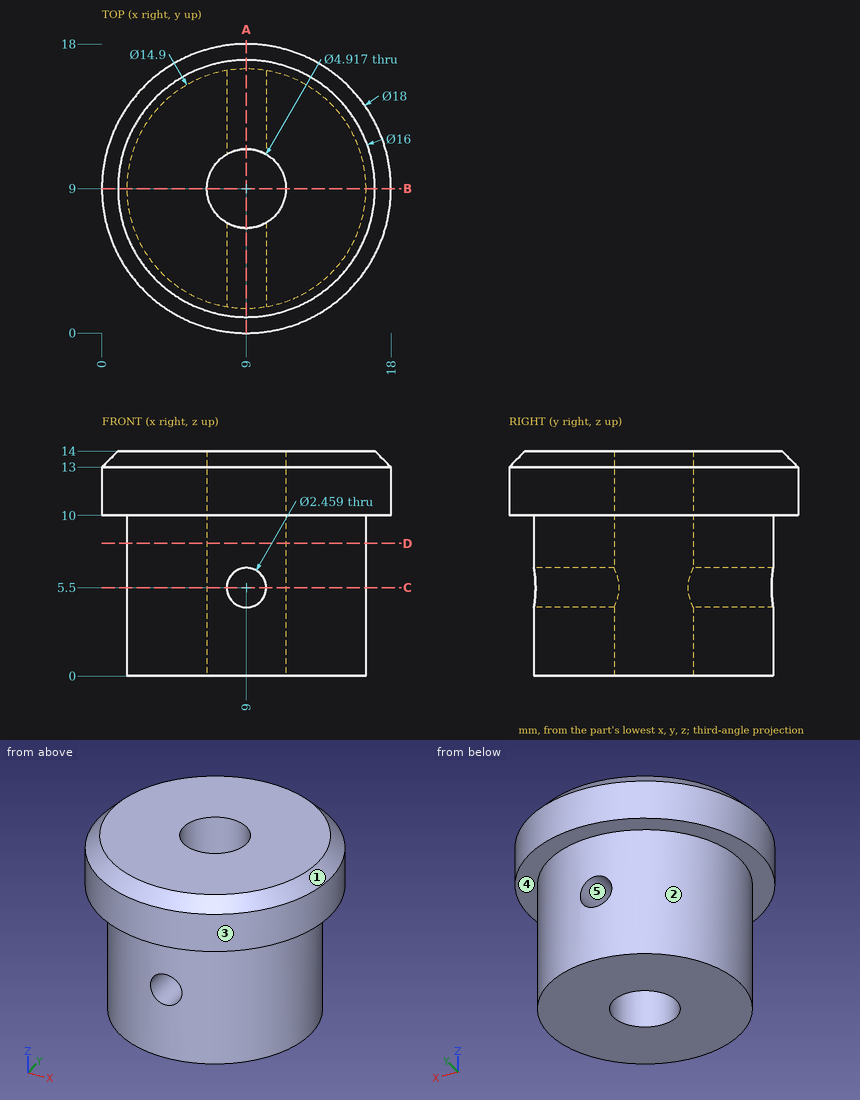
Here's the drawing with two shaded views (mm, measured from the low corner). I have some questions. A direction names the side the tool comes from. Coordinates: 2 decimals unless noted, no trailing zeros. Write each loop counter-clockwise with the first axis right and the second up, starting at its lowest first coordinate (ties: lowest second). Pieces come first, ordered by that corner, then holes. Notation, with made-up numbers: M 10.25,86 L 37.25,86 A26 cw 37.25,110 Z; hole C 21,32 d4. An arc over 180 degrees is marked long. Use one line per item in the form item = value.
Q1. If we section it at C-C (z = 5.5): Write out the boundary of the cut face in (x, y).
Model answer:
outline = M 7.77,1.65 L 7.77,6.87 A2.46 cw 7.77,11.13 L 7.77,16.35 A7.45 ccw Z; M 10.23,1.65 A7.45 ccw 10.23,16.35 L 10.23,11.13 A2.46 cw 10.23,6.87 Z
Q2. I need wall thicknesses on line 1 along Z through (x, y) = (9, 2.6); line 2 along Y through (x, z) = (9, 3); line 3 along Z through (x, y) = (13.25, 15.75). Which ranges of each line are inside material? Lowest first, please. Write a range as from..to.
Model answer:
line_1 = 0..4.27, 6.73..14
line_2 = 1.55..6.54, 11.46..16.45
line_3 = 10..14
Q3. If we section it at B-B (y = 9): Write out the boundary of the cut face in (x, z).
Model answer:
outline = M 0,10 L 1.55,10 L 1.55,0 L 6.54,0 L 6.54,14 L 1,14 L 0,13 Z; M 11.46,0 L 16.45,0 L 16.45,10 L 18,10 L 18,13 L 17,14 L 11.46,14 Z
Q4. For P1, Ø3, axis at x = 9, z = 5.5, coming from the +Y side; P2, Ø3, axis at x = 9, y = 9, coming from the -Z side; P3, Ø8, axis at y = 2.5, z = 4.5, coming from the +X side; P4, Ø1, axis at y = 3.5, z = 11, coming from the +X side, each with a flat end and sliding along its axis, tell me the tip position at first contact or that it passes through.
Model answer:
P1 = 16.45
P2 = through
P3 = 16.02
P4 = 16.48
Q5. We'd pull the mould along X, two halves only. Please class the marked faces 3, 4 and 5: +X half, -X half, draft (parallel to the pull), parting line (faces both ways), or undercut.
Model answer:
face_3 = parting line
face_4 = draft
face_5 = undercut
Q6. If we section it at A-A (x = 9): Write out the boundary of the cut face in (y, z), then the cut area to 3 significant figures.
Model answer:
outline = M 0,10 L 1.55,10 L 1.55,6.73 L 6.54,6.73 L 6.54,14 L 1,14 L 0,13 Z; M 1.55,0 L 6.54,0 L 6.54,4.27 L 1.55,4.27 Z; M 11.46,0 L 16.45,0 L 16.45,4.27 L 11.46,4.27 Z; M 11.46,6.73 L 16.45,6.73 L 16.45,10 L 18,10 L 18,13 L 17,14 L 11.46,14 Z
area = 127 mm^2
Q7. For the marked faces 1 and 2, which set-ups out of +Z, -Z, +X, -X, +Y, -Y let a thin tool reach every point of the face, with its end or its side?
Model answer:
face_1 = +Z
face_2 = -Z
Q8. If we section it at D-D (z = 8.25): Write out the boundary of the cut face in (x, y), then the cut area to 3 significant figures.
Model answer:
outline = C 9,9 d14.9; hole C 9,9 d4.92
area = 155 mm^2
